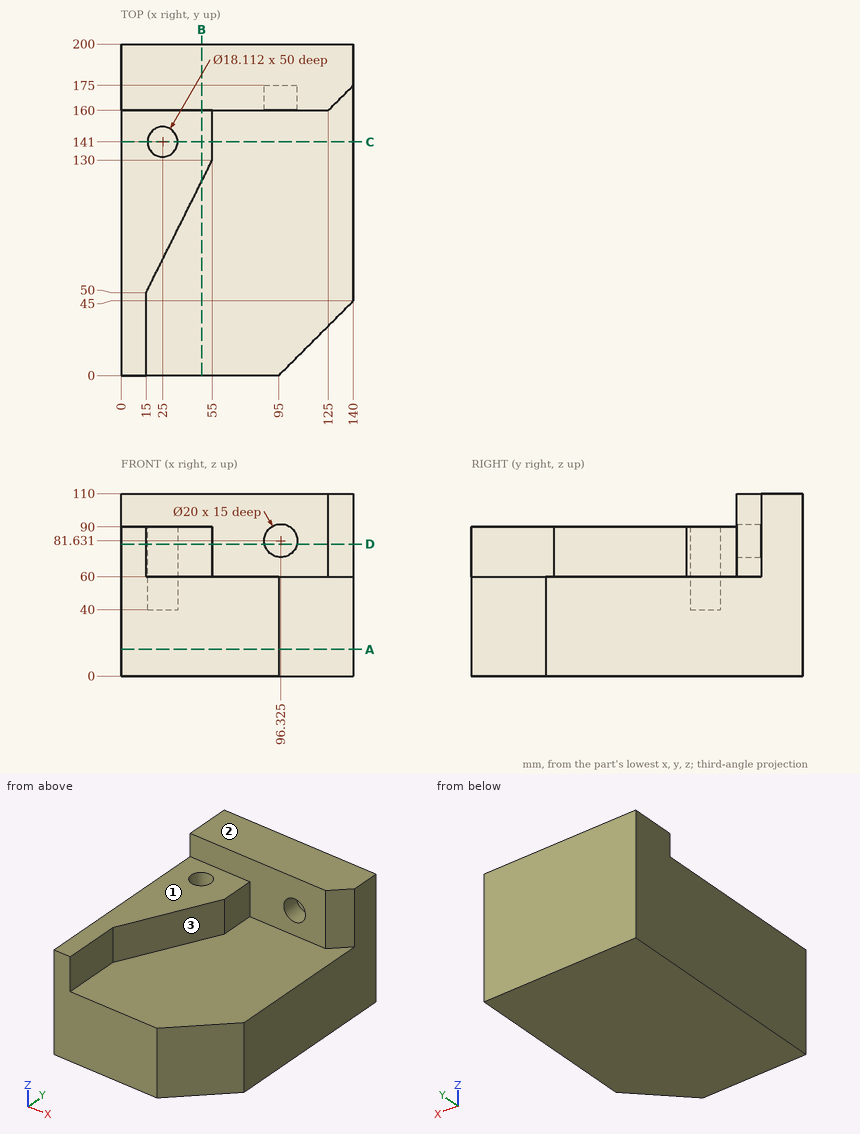
The drawing under review shows one solid part. Ordinate dimensions are in mm from its lowest x, y, z. A direction names the side the tool comes from. Give positions to 0.01 mm unless a question says otherwise; leave off trailing zeros. Order: outer loops, then holes, each group sorted by start corner. A loop starts at its lowest first (then second) coordinate and runs counter-clockwise, first axis right, second up. Notation, with made-up numbers: M -35,33.25 L -19,33.25 A19 ccw -19,46.25 Z; hole C -15.75,21.25 d11. An arc over 180 degrees is marked long. Answer in a Markdown table with one row per item. Add a question column.
1. Add section A-A on z = 16. State the section outline as (x, y) points, plus the area to 3 significant figures.
2. For pin 1 Ø3 at (x, y) = (56.5, 77.5) entering from +Z; pin 2 Ø20 at (x, y) = (28.5, 144.5) entering from +Z; pin 3 Ø18 at (x, z) = (96.32, 81.63) entering from -Y, all flat-tipped, find the tip position at first contact; note any pin that passes through.
3. Add section C-C on y = 141. State the section outline as (x, z) points.
4. Add section D-D on z = 79.5. State the section outline as (x, y) points (1 decimal), plus the area to 3 significant figures.
5. Add section B-B on x = 48.5. State the section outline as (y, z) points, plus the area to 3 significant figures.
6. To check wall thickness, follow line 1 along X through (y, z) = (141, 63.5); line 2 along Z through (x, y) = (103.5, 122.5); line 3 along Y through (x, z) = (102.5, 93). State the ranges of each line that lie inside material, in increasing order.
7. Machinability: for the marked faces 1, 2 and 3, which of the approach directions +Z, -Z, +X, -X, +Y, -Y give a long, thin tool a straight path to every point of the face, cutting with its end or side? Answer none if there is none.
The answers:
| question | item | result |
|---|---|---|
| 1 | outline | M 0,0 L 95,0 L 140,45 L 140,200 L 0,200 Z |
| 1 | area | 27,000 mm2 |
| 2 | pin 1 | z = 60 |
| 2 | pin 2 | z = 90 |
| 2 | pin 3 | y = 175 |
| 3 | outline | M 0,0 L 140,0 L 140,60 L 55,60 L 55,90 L 34.06,90 L 34.06,40 L 15.94,40 L 15.94,90 L 0,90 Z |
| 4 | outline | M 0,0 L 15,0 L 15,50 L 55,130 L 55,160 L 86.6,160 L 86.6,175 L 106.1,175 L 106.1,160 L 125,160 L 140,175 L 140,200 L 0,200 Z; hole C 25,141 d18.1 |
| 4 | area | 10,100 mm2 |
| 5 | outline | M 0,0 L 200,0 L 200,110 L 160,110 L 160,90 L 117,90 L 117,60 L 0,60 Z |
| 5 | area | 15,300 mm2 |
| 6 | line 1 | 0 to 15.94, 34.06 to 55 |
| 6 | line 2 | 0 to 60 |
| 6 | line 3 | 160 to 200 |
| 7 | face 1 | +Z, +X, -X, -Y |
| 7 | face 2 | +Z, +X, -X, +Y, -Y |
| 7 | face 3 | +Z, +X, -Y |
